Could you check a few things on this model? Use its own coordinates, in mm. A direction names the side the tool comes from. Coordinates: 2 decimals unless noted, no trailing zeros. Order: outer loops, then holes, each group sorted by start corner. A loop starts at its lowest first (then second) coordinate and runs counter-clockwise, first axis right, second up. Notation, with made-up numbers: (-28, 51) -> (-6, 51) arc R17 ccw to (-6, 62) -> close; hole circle Ø9 at (36.25, 11.5). An arc over 180 degrees is marked (long way). Put each result on its own line as item: value. Start each with the question number.
Q1. If we section it at D-D (x = -8.5): Please give me the cut outline in (y, z).
Q2. Please list where these lines run through material, in increasing order: line 1 along Z through (x, y) = (0, 6.75); line 2 along X through (y, z) = (7.25, 2.5).
Q3. For faces 1 (the face through (-1.42, 13, 3.92)), 2 (the face through (11.923, 5.972, -3.755)), which set-ups out of +Z, -Z, +X, -X, +Y, -Y let a thin tool reach every point of the face, with its end or its side?
Q4. If we section it at C-C (z = -2): Please give me the cut outline in (x, y), and give its area (3 significant figures).
Q5. Will these pins go through, and if not, where does the flat tip stop? pin 1 (1 mm diameter, centred on x = 6, y = 9, fed in from +Z); pin 2 (3 mm diameter, centred on y = 3, z = 9.5, fed in from -X); pin 3 (4 mm diameter, centred on x = 0, y = 10.5, fed in from -Z).
Q6. We'd pull the mould along Z, two halves only. Please class faces 3 (the face through (0, 4, 0)), 4 (the face through (-1.2, 9.6, -4.8)), 5 (the face through (23.75, 1.97, 0.09)), 6 (the face through (13.186, 1.972, 8.589)): +Z half, -Z half, draft (parallel to the pull), parting line (faces both ways), or undercut.
Q7. If we section it at A-A (x = 0): Please give me the cut outline in (y, z), and give its area (3 significant figures).
Q8. If we section it at B-B (x = 19.5): Please give me the cut outline in (y, z).
from build123d import *

# Parameters (mm, degrees)
SKETCH1_R           = 2.5
BOSS_EXTRUDE1_DEPTH = 4
SKETCH2_R           = 12.5
SKETCH2_R_2         = 10.5
EXTRUDE_THIN1_DEPTH = 4
SKETCH3_R           = 6
SKETCH3_R_2         = 4
EXTRUDE_THIN2_DEPTH = 9
SKETCH4_R           = 1.5
CUT_EXTRUDE1_DEPTH  = 31.254131949
CIRPATTERN1_COUNT   = 2
CIRPATTERN1_ANGLE   = 90


with BuildPart() as part:
    # Sketch1 → Boss-Extrude1 (new body)
    with BuildSketch(Plane(origin=(0, 0, 0), x_dir=(1, 0, 0), z_dir=(0, 1, 0))):
        with BuildLine():
            Line((20.660958904, 4.943407445), (5.917808219, 12.133818273))
            ThreePointArc((5.917808219, 12.133818273), (0, 13.5), (-5.917808219, 12.133818273))
            Line((-5.917808219, 12.133818273), (-20.660958904, 4.943407445))
            ThreePointArc((-20.660958904, 4.943407445), (-23.75, 0), (-20.660958904, -4.943407445))
            Line((-20.660958904, -4.943407445), (-5.917808219, -12.133818273))
            ThreePointArc((-5.917808219, -12.133818273), (0, -13.5), (5.917808219, -12.133818273))
            Line((5.917808219, -12.133818273), (20.660958904, -4.943407445))
            ThreePointArc((20.660958904, -4.943407445), (23.75, 0), (20.660958904, 4.943407445))
        make_face()
        with Locations(Location((18.25, 0, 0), (0, 0, 270))):
            Circle(SKETCH1_R, mode=Mode.SUBTRACT)
        with Locations(Location((-18.25, 0, 0), (0, 0, 90))):
            Circle(SKETCH1_R, mode=Mode.SUBTRACT)
    extrude(amount=BOSS_EXTRUDE1_DEPTH)

    # Sketch2 → Extrude-Thin1 (add)
    with BuildSketch(Plane(origin=(0, 4, 0), x_dir=(1, 0, 0), z_dir=(0, 1, 0))):
        Circle(SKETCH2_R)
        Circle(SKETCH2_R_2, mode=Mode.SUBTRACT)
    extrude(amount=EXTRUDE_THIN1_DEPTH)

    # Sketch3 → Extrude-Thin2 (add)
    with BuildSketch(Plane(origin=(0, 4, 0), x_dir=(1, 0, 0), z_dir=(0, 1, 0))):
        Circle(SKETCH3_R)
        Circle(SKETCH3_R_2, mode=Mode.SUBTRACT)
    extrude(amount=EXTRUDE_THIN2_DEPTH)

    # Sketch4 → Cut-Extrude1 (cut, symmetric)
    with BuildSketch(Plane.XY):
        with Locations((0, 10.5)):
            Circle(SKETCH4_R)
    cut_extrude1 = extrude(amount=CUT_EXTRUDE1_DEPTH, both=True, mode=Mode.SUBTRACT)

    # CirPattern1: Cut-Extrude1 ×2 about axis
    cirpattern1_axis = Axis((0, 13, 0), (0, 1, 0))
    for i in range(1, CIRPATTERN1_COUNT):
        add(cut_extrude1.rotate(cirpattern1_axis, i * CIRPATTERN1_ANGLE / (CIRPATTERN1_COUNT - 1)), mode=Mode.SUBTRACT)


solid = part.part
The answers:
1. outline: (0, -10.87) -> (4, -10.87) -> (4, -9.17) -> (8, -9.17) -> (8, -6.16) -> (4, -6.16) -> (4, 6.16) -> (8, 6.16) -> (8, 9.17) -> (4, 9.17) -> (4, 10.87) -> (0, 10.87) -> close
2. line 1: -12.5 to -10.5, -6 to -4, 4 to 6, 10.5 to 12.5
2. line 2: -12.25 to -10.2, -5.45 to -3.12, 3.12 to 5.45, 10.2 to 12.25
3. face 1: +Z, -Z, +X, -X, +Y
3. face 2: +Y
4. outline: (-23.37, 0) -> (-19.75, 0) -> (-19.75, 4) -> (-23.37, 4) -> close; (-16.75, 0) -> (16.75, 0) -> (16.75, 4) -> (12.34, 4) -> (12.34, 8) -> (10.31, 8) -> (10.31, 4) -> (5.66, 4) -> (5.66, 13) -> (3.46, 13) -> (3.46, 4) -> (-3.46, 4) -> (-3.46, 13) -> (-5.66, 13) -> (-5.66, 4) -> (-10.31, 4) -> (-10.31, 8) -> (-12.34, 8) -> (-12.34, 4) -> (-16.75, 4) -> close; (19.75, 0) -> (23.37, 0) -> (23.37, 4) -> (19.75, 4) -> close
4. area: 219 mm^2
5. pin 1: z = 2.4
5. pin 2: x = -14.39
5. pin 3: z = -6
6. face 3: undercut
6. face 4: draft
6. face 5: parting line
6. face 6: +Z half
7. outline: (0, -13.5) -> (4, -13.5) -> (4, -12.5) -> (8, -12.5) -> (8, -10.5) -> (4, -10.5) -> (4, -6) -> (9, -6) -> (9, -4) -> (4, -4) -> (4, 4) -> (9, 4) -> (9, 6) -> (4, 6) -> (4, 10.5) -> (8, 10.5) -> (8, 12.5) -> (4, 12.5) -> (4, 13.5) -> (0, 13.5) -> close; (12, -6) -> (13, -6) -> (13, -4) -> (12, -4) -> close; (12, 4) -> (13, 4) -> (13, 6) -> (12, 6) -> close
7. area: 148 mm^2
8. outline: (0, -5.51) -> (4, -5.51) -> (4, -2.17) -> (0, -2.17) -> close; (0, 2.17) -> (4, 2.17) -> (4, 5.51) -> (0, 5.51) -> close
